Verification items for the finished model (mm, model axes). Round coordinates to 2 decimals unless told otherwise and drop trailing zeros. Loops run counter-clockwise (first coordinate to the right, second up) from the corner with the lowest first, then second, coordinate; pieces in that order, holes last. Notation, with made-up numbers: M 3,-0.75 L 24,-0.75 A24 ccw 24,23.25 Z; hole C -27,39 d11. An arc over 180 degrees is marked long. One line per item, written item: value.
from build123d import *

# Parameters (mm, degrees)
BOSS_EXTRUDE1_DEPTH = 3
FILLET1_R           = 10
FILLET2_R           = 1
FILLET3_R           = 1.5
FILLET4_R           = 4
FILLET5_R           = 4


with BuildPart() as part:
    # Sketch2 → Boss-Extrude1 (new body)
    with BuildSketch(Plane(origin=(0, 0, 0), x_dir=(1, 0, 0), z_dir=(0, 1, 0))):
        with BuildLine():
            Line((-42.5, 9.815250458), (-40.2, 13.848552856))
            ThreePointArc((-40.2, 13.848552856), (-31.616402931, 19.380516515), (-21.88, 22.46))
            ThreePointArc((-21.88, 22.46), (-15.087159026, 34.642704233), (-4.89, 44.16))
            Line((-4.89, 44.16), (-8.851038754, 46.435359195))
            Line((-8.851038754, 46.435359195), (-10.31, 48.433697347))
            Line((-10.31, 48.433697347), (-9.719569356, 51.28656851))
            Line((-9.719569356, 51.28656851), (-4.45, 52.03))
            Line((-4.45, 52.03), (2.1, 44.53))
            Line((2.1, 44.53), (35.22, 47.35))
            ThreePointArc((35.22, 47.35), (39.1087714, 53.552611798), (45.450837647, 49.895682508))
            Line((45.450837647, 49.895682508), (49.271682555, 36.649721013))
            ThreePointArc((49.271682555, 36.649721013), (51.113757972, 35.62), (52.162431436, 37.451352279))
            Line((52.162431436, 37.451352279), (49.298477535, 47.38))
            Line((49.298477535, 47.38), (47.49564271, 53.63))
            Line((47.49564271, 53.63), (59.07164271, 53.63))
            ThreePointArc((59.07164271, 53.63), (60.57164271, 55.13), (59.07164271, 56.63))
            Line((59.07164271, 56.63), (48.07164271, 56.63))
            Line((48.07164271, 56.63), (48.010812194, 60.48))
            ThreePointArc((48.010812194, 60.48), (62.895920888, 72.4), (77.21, 59.8))
            ThreePointArc((77.21, 59.8), (75.464062366, 48.951036242), (71.72, 38.62))
            ThreePointArc((71.72, 38.62), (64.699564013, 29.762620869), (54.32, 25.29))
            Line((54.32, 25.29), (12.44, 30.35))
            ThreePointArc((12.44, 30.35), (-2.155765073, 27.757228529), (-12.82, 17.46))
            Line((-12.82, 17.46), (-7.923093172, 14.42))
            Line((-7.923093172, 14.42), (4.26, 16.67))
            Line((4.26, 16.67), (10.264967392, 14.82186735))
            Line((10.264967392, 14.82186735), (15.68118928, 17.321714129))
            Line((15.68118928, 17.321714129), (26.105067381, 16.67))
            Line((26.105067381, 16.67), (27.5, 15.12))
            ThreePointArc((27.5, 15.12), (27.256062178, 10.796585791), (24.812537217, 7.22158903))
            Line((24.812537217, 7.22158903), (22.269740859, 7.646334739))
            Line((22.269740859, 7.646334739), (23.205269456, 10.857431213))
            Line((23.205269456, 10.857431213), (19.255161489, 11.297641869))
            Line((19.255161489, 11.297641869), (11.827625236, 7.22158903))
            Line((11.827625236, 7.22158903), (9.25, 9.1))
            Line((9.25, 9.1), (0.278765895, 9.8))
            Line((0.278765895, 9.8), (0, 7.298571725))
            Line((0, 7.298571725), (-7.923093172, 8.181542538))
            ThreePointArc((-7.923093172, 8.181542538), (-9.58, 6.856906829), (-8.255364291, 5.2))
            Line((-8.255364291, 5.2), (0, 4.28))
            Line((0, 4.28), (0, 0))
            Line((0, 0), (-20.44, 0))
            Line((-20.44, 0), (-23.89, 13.229016126))
            Line((-23.89, 13.229016126), (-25.72, 14.58))
            Line((-25.72, 14.58), (-29.87882635, 11.312892327))
            Line((-29.87882635, 11.312892327), (-33.582044966, 9.115250458))
            Line((-33.582044966, 9.115250458), (-36.680656461, 12.703691255))
            Line((-36.680656461, 12.703691255), (-42.5, 9.815250458))
        make_face()
    extrude(amount=BOSS_EXTRUDE1_DEPTH)

    # Fillet1
    fillet1_edges = [part.edges().sort_by_distance(p)[0] for p in [
        (-7.923093172, 1.5, -14.42),
    ]]
    fillet(fillet1_edges, radius=FILLET1_R)

    # Fillet2
    fillet2_edges = [part.edges().sort_by_distance(p)[0] for p in [
        (-42.5, 1.5, -9.815250458),
    ]]
    fillet(fillet2_edges, radius=FILLET2_R)

    # Fillet3
    fillet3_edges = [part.edges().sort_by_distance(p)[0] for p in [
        (4.26, 1.5, -16.67),
        (26.105067381, 1.5, -16.67),
        (27.5, 1.5, -15.12),
        (24.812537217, 1.5, -7.22158903),
        (23.205269456, 1.5, -10.857431213),
        (19.255161489, 1.5, -11.297641869),
        (11.827625236, 1.5, -7.22158903),
        (9.25, 1.5, -9.1),
        (0.278765895, 1.5, -9.8),
        (0, 1.5, 0),
        (-20.44, 1.5, 0),
        (-23.89, 1.5, -13.229016126),
        (-25.72, 1.5, -14.58),
        (-21.88, 1.5, -22.46),
        (-4.89, 1.5, -44.16),
        (-4.45, 1.5, -52.03),
        (2.1, 1.5, -44.53),
        (35.22, 1.5, -47.35),
    ]]
    fillet(fillet3_edges, radius=FILLET3_R)

    # Fillet4
    fillet4_edges = [part.edges().sort_by_distance(p)[0] for p in [
        (-33.582044966, 1.5, -9.115250458),
        (-10.31, 1.5, -48.433697347),
    ]]
    fillet(fillet4_edges, radius=FILLET4_R)

    # Fillet5
    fillet5_edges = [part.edges().sort_by_distance(p)[0] for p in [
        (10.264967392, 1.5, -14.82186735),
        (15.68118928, 1.5, -17.321714129),
    ]]
    fillet(fillet5_edges, radius=FILLET5_R)


solid = part.part
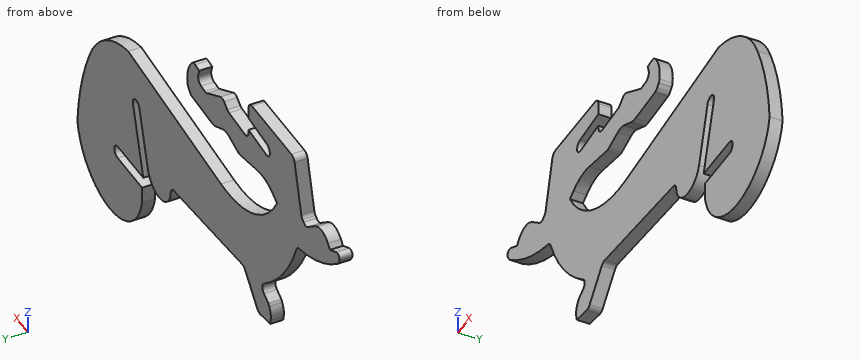
(1) Depth check by flat-ended pin: pin 1 Ø0.9 at (x, y) = (54.5, 1) entering from -Z; pin 2 Ø1 at (y, z) = (2, -45.5) entering from +X; pin 3 Ø1.5 at (x, y) = (56, 1.5) entering from +Z. Enter the tip coordinate at first touch or a pass-through.
Completed:
pin 1: stops at z = -70.31
pin 2: stops at x = 74.62
pin 3: stops at z = -25.46
(2) Thickness scan on L1, parallel to X at y = 1.35, z = -50; L2, parallel to X at y = 0.95, z = -50.5; L3, parallel to Z at x = -3.5, y = 2.45. Record the ranges inside material, lowest first. Write a range as from..to.
Completed:
L1: x = -9.98..-2.68, 35.35..45.42, 48.54..75.73
L2: x = -9.88..-3.11, 35.53..45.24, 48.4..75.84
L3: z = -50.94..-27.02, -15.24..-7.69, -4.67..0
(3) Sectioned sample at B-B on x = 31. Enter the section's corners in (y, z).
Completed:
outline: M 0,-46.99 L 3,-46.99 L 3,-28.11 L 0,-28.11 Z
(4) Sectioned sample at A-A on z = -27. Enter the section's corners in (x, y), and give its area (3 significant figures).
Completed:
outline: M -19.92,0 L -3.53,0 L -3.53,3 L -19.92,3 Z; M 40.17,0 L 60.06,0 L 60.06,3 L 40.17,3 Z
area: 109 mm^2
(5) Sectioned sample at C-C on z = -55.13. Enter the section's corners in (x, y).
Completed:
outline: M 60.57,0 L 76.71,0 L 76.71,3 L 60.57,3 Z
